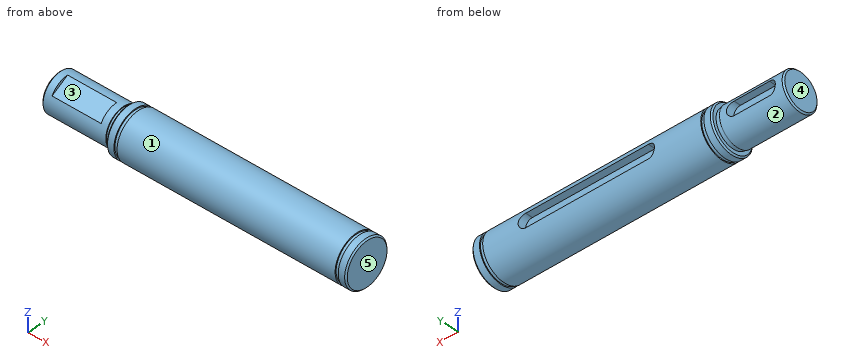
Autodesk Inventor part; units mm, degrees
ref_plane "to_c_ring_2_XY" through (28.425, 0, 0) normal (1, 0, 0) x (0, 0, 1)
ref_plane "to_c_ring_2_YZ" through (28.425, 0, 0) normal (0, 0, 1) x (0, -1, 0)
ref_plane "to_c_ring_2_ZX" through (28.425, 0, 0) normal (0, -1, 0) x (1, 0, 0)
sketch "Sketch_1" plane through (0, 0, 0) normal (0, 0, 1) x (1, 0, 0)
  line L0 (113, 0) -> (0, 0)
  line L1 (0, 0) -> (0, 6.5)
  line L2 (0, 6.5) -> (0.5, 7)
  line L3 (0.5, 7) -> (25, 7)
  line L4 (25, 7) -> (25, 8)
  line L5 (25, 8) -> (25.5, 8.5)
  line L6 (25.5, 8.5) -> (112.5, 8.5)
  line L7 (112.5, 8.5) -> (113, 8)
  line L8 (113, 8) -> (113, 0)
  line L9 (113, 0) -> (0, 0)
revolve "Revolution1" add sketch "Sketch_1" angle 360 about axis through (113, 0, 0) along (1, 0, 0)
sketch "Sketch_2" plane through (0, 0, 0) normal (0, 0, 1) x (1, 0, 0)
  line L0 (50, 0) -> (-50, 0)
  line L1 (23.5, 21) -> (23.5, 6.7)
  line L2 (23.5, 6.7) -> (25, 6.7)
  line L3 (25, 6.7) -> (25, 21)
  line L4 (25, 21) -> (23.5, 21)
revolve "Revolution2" cut sketch "Sketch_2" angle 360 about axis through (50, 0, 0) along (1, 0, 0)
sketch "Sketch_15" plane through (0, 0, 0) normal (0, 0, 1) x (1, 0, 0)
  line L0 (50, 0) -> (-50, 0)
  line L1 (27.85, 25.1) -> (27.85, 8.1)
  line L2 (27.85, 8.1) -> (29, 8.1)
  line L3 (29, 8.1) -> (29, 25.1)
  line L4 (29, 25.1) -> (27.85, 25.1)
revolve "Revolution3" cut sketch "Sketch_15" angle 360 about axis through (50, 0, 0) along (1, 0, 0)
sketch "Sketch_16" plane through (0, 0, 0) normal (0, 0, 1) x (1, 0, 0)
  line L0 (113, 0) -> (-50, 0)
  line L1 (109, 25.1) -> (109, 8.1)
  line L2 (109, 8.1) -> (110.15, 8.1)
  line L3 (110.15, 8.1) -> (110.15, 25.1)
  line L4 (110.15, 25.1) -> (109, 25.1)
revolve "Revolution4" cut sketch "Sketch_16" angle 360 about axis through (113, 0, 0) along (1, 0, 0)
sketch "Sketch_20" plane through (0, 8.5, 0) normal (0, 1, 0) x (1, 0, 0)
  arc A0 (48.5, 2.5) -> (48.5, -2.5) centre (48.5, 0) ccw
  line L0 (48.5, -2.5) -> (93.5, -2.5)
  arc A1 (93.5, -2.5) -> (93.5, 2.5) centre (93.5, 0) ccw
  line L1 (93.5, 2.5) -> (48.5, 2.5)
extrude "Extrusion1" cut sketch "Sketch_20" against normal blind 3
sketch "Sketch_21" plane through (0, 7, 0) normal (0, 1, 0) x (1, 0, 0)
  arc A0 (5.5, 2.5) -> (5.5, -2.5) centre (5.5, 0) ccw
  line L0 (5.5, -2.5) -> (18.5, -2.5)
  arc A1 (18.5, -2.5) -> (18.5, 2.5) centre (18.5, 0) ccw
  line L1 (18.5, 2.5) -> (5.5, 2.5)
extrude "Extrusion2" cut sketch "Sketch_21" against normal blind 3
sketch "Sketch_63" plane through (3, 0, 0) normal (1, 0, 0) x (0, 0, -1)
  line L0 (-13.0622, 8.6244) -> (0.9378, -15.6244)
  line L1 (0.9378, -15.6244) -> (1.8038, -15.1244)
  line L2 (1.8038, -15.1244) -> (-12.1962, 9.1244)
  line L3 (-12.1962, 9.1244) -> (-13.0622, 8.6244)
extrude "Extrusion3" cut sketch "Sketch_63" along normal blind 18
ref_plane "to_c_ring_2_XY" through (28.425, 0, 0) normal (1, 0, 0) x (0, 0, 1)
ref_plane "to_c_ring_2_YZ" through (28.425, 0, 0) normal (0, 0, 1) x (0, -1, 0)
ref_plane "to_c_ring_2_ZX" through (28.425, 0, 0) normal (0, -1, 0) x (1, 0, 0)
ref_plane "to_c_ring_3_XY" through (109.575, 0, 0) normal (1, 0, 0) x (0, 0, 1)
ref_plane "to_c_ring_3_YZ" through (109.575, 0, 0) normal (0, 0, 1) x (0, -1, 0)
ref_plane "to_c_ring_3_ZX" through (109.575, 0, 0) normal (0, -1, 0) x (1, 0, 0)
properties part number "KZBN17-113-P14-LA25-TC4-TB4-KB21-HB50-ZA3-HA18-AA120_b" material "Stainless Steel"
Geometry check sheet. Reference: the model listing, model coordinates, mm. Face numbers are marked on the shaded views. A direction names the side the tool comes from. Give positions to 0.01 mm unless a question says otherwise; leave off trailing zeros. Loops run counter-clockwise (first coordinate to the right, second up) from the corner with the lowest first, then second, coordinate; pieces in that order, holes last. Notation, with made-up numbers: (15, -36) -> (51, -36) arc R8 ccw to (51, -32) -> close; hole circle Ø8 at (-36.5, 38.25). An arc over 180 degrees is marked (long way). Answer in a Markdown table with one row per item. Add a question column.
1) Set-up check for the marked faces 1 and 2: record each of +Z, -Z, +X, -X, +Y, -Y from which the full face is reachable in a straight line by a thin tool's end or side.
2) Draft check along X on the marked faces 3, 4 and 5. Enter one of: pulls with the +X half, pulls with the -X half, needs draft (parallel to the pull), parting line crosses it, or undercut.
3) Material ranges on probe 1 along X at (y, z) = (-6.25, -5.25); probe 2 along X at (y, z) = (-6, -4.75); probe 3 along Y at (x, z) = (38.5, -0.5), recorded low to high. Write a range as from..to.
4) Gauge pin test, flat ends, axial feed: P1, Ø4, axis at x = 64.5, z = -1, coming from the +Y side; P2, Ø6, axis at x = 80.5, y = -6, coming from the -Z side; P3, Ø1.5, axis at x = 12.5, z = -1, coming from the +Y side. Record the tip position at first contact, or that the pin passes through.
5) Cross-section at A-A on x = 53. Record the boundary of the cut face in (y, z).
Outcome:
| question | item | result |
|---|---|---|
| 1 | face 1 | +X, -X |
| 1 | face 2 | -X |
| 2 | face 3 | undercut |
| 2 | face 4 | pulls with the -X half |
| 2 | face 5 | pulls with the +X half |
| 3 | probe 1 | x = 25.16..27.85, 29..109, 110.15..112.84 |
| 3 | probe 2 | x = 25..113 |
| 3 | probe 3 | y = -8.49..8.49 |
| 4 | P1 | stops at y = 8.12 |
| 4 | P2 | stops at z = -7.95 |
| 4 | P3 | stops at y = 4 |
| 5 | outline | (5.5, -2.5) -> (5.5, 2.5) -> (8.12, 2.5) arc R8.5 ccw (long way) to (8.12, -2.5) -> close |
